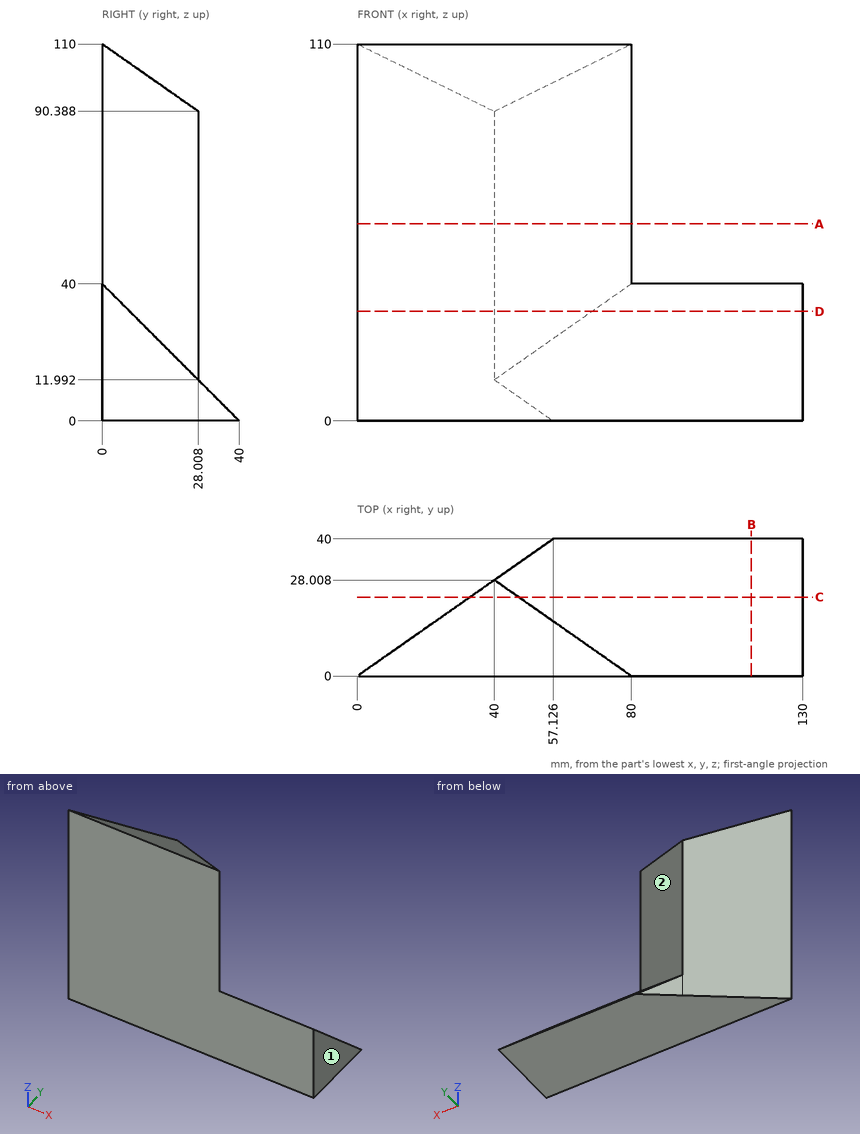
Study the drawing (mm; zero at the part's minimum x, y, z) and answer. A direction names the side the tool comes from. Give positions to 0.01 mm unless a question says otherwise; leave off trailing zeros. Write each loop counter-clockwise with the first axis right and the second up, starting at its lowest first coordinate (ties: lowest second). Pieces come first, ordered by that corner, then holes. Notation, with made-up numbers: (-26.75, 85) - (23.25, 85) arc R4 cw to (23.25, 90) - close; hole circle Ø8 at (46.5, 55). An arc over 180 degrees is marked (long way). Use a Markdown table: item, result.
1. Find the intervals of material crossed by probe 1 along Z at (x, y) = (66, 12); probe 2 along Y at (x, z) = (26.5, 34.5) (1 decimal); probe 3 along X at (y, z) = (18.5, 35), in increasing order. Write a range as from..to.
Values follow:
| item | result |
|---|---|
| probe 1 | z = 0..28 |
| probe 2 | y = 0..18.6 |
| probe 3 | x = 26.42..53.58 |
2. Section D-D on z = 32 is taken. Write down the section's boundary in (x, y) (1 decimal).
Values follow:
| item | result |
|---|---|
| outline | (0, 0) - (130, 0) - (130, 8) - (68.6, 8) - (40, 28) - close |
3. Section C-C on y = 23 is taken. Write down the section's boundary in (x, z) (1 decimal), plus the area to 3 significant figures.
Values follow:
| item | result |
|---|---|
| outline | (32.8, 0) - (130, 0) - (130, 17) - (47.2, 17) - (47.2, 93.9) - (32.8, 93.9) - close |
| area | 2,750 mm² |
4. Section A-A on z = 57.5 is taken. Write down the section's boundary in (x, y), plus the area to 3 significant figures.
Values follow:
| item | result |
|---|---|
| outline | (0, 0) - (80, 0) - (40, 28.01) - close |
| area | 1,120 mm² |
5. Section B-B on x = 115 is taken. Write down the section's boundary in (y, z), plus the area to 3 significant figures.
Values follow:
| item | result |
|---|---|
| outline | (0, 0) - (40, 0) - (0, 40) - close |
| area | 800 mm² |
6. Each of these flat-tipped pins is pushed along its axis until it touches: P1, Ø10, axis at x = 90.5, y = 31, coming from the +Z side; P2, Ø6, axis at y = 15, z = 31.5, coming from the +X side; P3, Ø1, axis at y = 8.5, z = 98, coming from the -X side (1 decimal). Where does it stop, or does it pass through?
Values follow:
| item | result |
|---|---|
| P1 | stops at z = 14 |
| P2 | stops at x = 62.86 |
| P3 | stops at x = 11.4 |
7. A tool of negligible diameter and unlimited length cuts with its end or side. For the marked faces 1 and 2, from which of +Z, -Z, +X, -X, +Y, -Y can it reach the whole face along a straight path? Write none if from no direction.
Values follow:
| item | result |
|---|---|
| face 1 | +Z, -Z, +X, +Y, -Y |
| face 2 | +Z, +X, +Y |
